Read the model definition and answer for the solid it produces. Units are mm, in the model's axes. A direction names the side the tool comes from. Give positions to 0.01 mm unless a question says otherwise; leave off trailing zeros. Loops run counter-clockwise (first coordinate to the right, second up) from the corner with the lowest first, then second, coordinate; pieces in that order, holes last. Notation, with made-up numbers: (15.25, 23) - (52.25, 23) arc R18 ccw to (52.25, 58) - close; hole circle Ø3 at (57.5, 44). An arc over 180 degrees is marked (long way). Put each result on its own line as item: value. Start each with the question number.
1. Given pin 1 Ø12 at (x, z) = (-4.5, 12) entering from -Y; pin 2 Ø4 at (x, z) = (-8.5, 9.5) entering from -Y; pin 3 Ø5 at (y, z) = (6, 8) entering from +X; pin 4 Ø2 at (x, y) = (37.5, -1.5) entering from -Z, each flat-ended and moving along its own axis, determine where each tip first touches the part or whether it passes through.
2. For a pull along Z with two mould halves and no side action, classify faces 1 (the cylindrical face through (0.426, -1.475, 1.872)), 2 (the cylindrical face through (20.06, 7.95, 8.37)), 3 (the flat face through (-50.8, 0, -5)) as released by +Z, released by -Z, zero draft, split by the parting line, or undercut.
3. A cutting plane is placed at D-D, the plane x = 0. Determine the outline of the cut face in (y, z) (3 decimals), plus the area to 3 significant figures.
4. Consider L1, parallel to Z at x = -18.4, y = 7.75; L2, parallel to X at y = -2.5, z = -4; L3, parallel to Z at x = -30.5, y = -8.5. Determine where each line is inside the solid, lowest interval first. Write a range as from..to.
5. For faces 4 (the cylindrical face through (-47.793, 10.01, -4.998)), 5 (the cylindrical face through (47.793, 10.01, -4.998)), 6 (the flat face through (-25.4, 7, 10)), determine the directions among +Z, -Z, +X, -X, +Y, -Y from which every point of the face is accessible in a straight line to the end or side of a thin tool.
6. A cutting plane is placed at B-B, the plane y = 0. Determine the outline of the cut face in (x, z) (3 decimals), plus the area to 3 significant figures.
7. A cutting plane is placed at C-C, the plane z = 8. Determine the outline of the cut face in (x, y) (3 decimals), plus the area to 3 significant figures.
8. A cutting plane is placed at A-A, the plane x = 38.1. Determine the outline of the cut face in (y, z) (3 decimals), plus the area to 3 significant figures.
```python
from build123d import *

# Parameters (mm, degrees)
SKETCH1_W                = 101.6
SKETCH1_H                = 25.4
BOSS_EXTRUDE1_DEPTH      = 10
SKETCH4_W                = 50.8
SKETCH4_H                = 20
BOSS_EXTRUDE2_DEPTH      = 10
BOSS_EXTRUDE4_DEPTH      = 50.8
BOSS_EXTRUDE4_DEPTH_BACK = 50.8
SKETCH9_W                = 25.4
SKETCH9_H                = 20
CUT_EXTRUDE4_DEPTH       = 61.214616166
FILLET1_R                = 10
CUT_EXTRUDE1_REACH       = 58.726
SKETCH5_R                = 3.175
SKETCH5_R_2              = 1.7
CUT_EXTRUDE2_REACH       = 58.283
SKETCH6_R                = 3.175
FILLET2_R                = 10
CUT_EXTRUDE3_REACH       = 58.726
SKETCH7_R                = 6
SKETCH7_R_2              = 3
FILLET3_R                = 5
FILLET4_R                = 5


with BuildPart() as part:
    # Sketch1 → Boss-Extrude1 (new body)
    with BuildSketch(Plane.XY):
        Rectangle(SKETCH1_W, SKETCH1_H)
    extrude(amount=-BOSS_EXTRUDE1_DEPTH)

    # Sketch4 → Boss-Extrude2 (add)
    with BuildSketch(Plane(origin=(0, 12.7, 0), x_dir=(1, 0, 0), z_dir=(0, 1, 0))):
        with Locations((0, -10)):
            Rectangle(SKETCH4_W, SKETCH4_H)
    extrude(amount=-BOSS_EXTRUDE2_DEPTH)

    # Sketch8 → Boss-Extrude4 (add, two sides: drawn at the far end of the back side and taken through both)
    with BuildSketch(Plane(origin=(0, 0, 0), x_dir=(0, 0, -1), z_dir=(1, 0, 0)).offset(-BOSS_EXTRUDE4_DEPTH_BACK)):
        Polygon((10, 12.7), (-20, 13.680158925), (-20, 12.7), align=None)
    extrude(amount=BOSS_EXTRUDE4_DEPTH + BOSS_EXTRUDE4_DEPTH_BACK)

    # Sketch9 → Cut-Extrude4 (cut, through all)
    with BuildSketch(Plane.XZ.offset(-12.7)):
        with Locations((-38.1, 10)):
            Rectangle(SKETCH9_W, SKETCH9_H)
        with Locations((38.1, 10)):
            Rectangle(SKETCH9_W, SKETCH9_H)
    extrude(amount=-CUT_EXTRUDE4_DEPTH, mode=Mode.SUBTRACT)

    # Fillet1
    fillet1_edges = [part.edges().sort_by_distance(p)[0] for p in [
        (0, 2.7, 0),
    ]]
    fillet(fillet1_edges, radius=FILLET1_R)

    # Cut-Extrude1: up to this plane
    cut_extrude1_end = Plane(origin=(50.8, 12.7, -10), z_dir=(0, -0.9994666982985511, 0.03265454014671021))
    # Sketch5 → Cut-Extrude1 (cut, up to the surface)
    with BuildSketch(Plane(origin=(0, 2.7, 0), x_dir=(1, 0, 0), z_dir=(0, 1, 0)), mode=Mode.PRIVATE) as cut_extrude1_sk1:
        with Locations(Location((0, -8, 0), (0, 0, 90))):
            Circle(SKETCH5_R)
    cut_extrude1_tool1 = split(extrude(cut_extrude1_sk1.sketch, amount=CUT_EXTRUDE1_REACH, mode=Mode.PRIVATE), bisect_by=cut_extrude1_end, keep=Keep.BOTH, mode=Mode.PRIVATE)
    add(cut_extrude1_tool1.solids().sort_by_distance((0, 2.7, 8))[0], mode=Mode.SUBTRACT)
    # Sketch5 → Cut-Extrude1 (cut, up to the surface)
    with BuildSketch(Plane(origin=(0, 2.7, 0), x_dir=(1, 0, 0), z_dir=(0, 1, 0)), mode=Mode.PRIVATE) as cut_extrude1_sk2:
        with Locations(Location((-18.4, -8, 0), (0, 0, 90))):
            Circle(SKETCH5_R_2)
    cut_extrude1_tool2 = split(extrude(cut_extrude1_sk2.sketch, amount=CUT_EXTRUDE1_REACH, mode=Mode.PRIVATE), bisect_by=cut_extrude1_end, keep=Keep.BOTH, mode=Mode.PRIVATE)
    add(cut_extrude1_tool2.solids().sort_by_distance((-18.4, 2.7, 8))[0], mode=Mode.SUBTRACT)
    # Sketch5 → Cut-Extrude1 (cut, up to the surface)
    with BuildSketch(Plane(origin=(0, 2.7, 0), x_dir=(1, 0, 0), z_dir=(0, 1, 0)), mode=Mode.PRIVATE) as cut_extrude1_sk3:
        with Locations(Location((18.4, -8, 0), (0, 0, 90))):
            Circle(SKETCH5_R_2)
    cut_extrude1_tool3 = split(extrude(cut_extrude1_sk3.sketch, amount=CUT_EXTRUDE1_REACH, mode=Mode.PRIVATE), bisect_by=cut_extrude1_end, keep=Keep.BOTH, mode=Mode.PRIVATE)
    add(cut_extrude1_tool3.solids().sort_by_distance((18.4, 2.7, 8))[0], mode=Mode.SUBTRACT)

    # Sketch6 → Cut-Extrude2 (cut, up to next)
    with BuildSketch(Plane.XY, mode=Mode.PRIVATE) as cut_extrude2_sk1:
        with Locations((-38.1, 0)):
            Circle(SKETCH6_R)
    cut_extrude2_tool1 = extrude(cut_extrude2_sk1.sketch, amount=-CUT_EXTRUDE2_REACH, mode=Mode.PRIVATE) & part.part
    # Sketch6 → Cut-Extrude2 (cut, up to next)
    with BuildSketch(Plane.XY, mode=Mode.PRIVATE) as cut_extrude2_sk2:
        with Locations(Location((38.1, 0, 0), (0, 0, 180))):
            Circle(SKETCH6_R)
    cut_extrude2_tool2 = extrude(cut_extrude2_sk2.sketch, amount=-CUT_EXTRUDE2_REACH, mode=Mode.PRIVATE) & part.part
    add(cut_extrude2_tool1.solids().sort_by_distance((-38.1, 0, 0))[0], mode=Mode.SUBTRACT)
    add(cut_extrude2_tool2.solids().sort_by_distance((38.1, 0, 0))[0], mode=Mode.SUBTRACT)

    # Fillet2
    fillet2_edges = [part.edges().sort_by_distance(p)[0] for p in [
        (-50.8, 12.863359821, -5),
        (50.8, 12.863359821, -5),
        (50.8, -12.7, -5),
        (-50.8, -12.7, -5),
    ]]
    fillet(fillet2_edges, radius=FILLET2_R)

    # Sketch7 → Cut-Extrude3 (cut, up to next)
    with BuildSketch(Plane.XZ.offset(-2.7), mode=Mode.PRIVATE) as cut_extrude3_sk1:
        with Locations((0, 8)):
            Circle(SKETCH7_R)
    cut_extrude3_tool1 = extrude(cut_extrude3_sk1.sketch, amount=CUT_EXTRUDE3_REACH, mode=Mode.PRIVATE) & part.part
    # Sketch7 → Cut-Extrude3 (cut, up to next)
    with BuildSketch(Plane.XZ.offset(-2.7), mode=Mode.PRIVATE) as cut_extrude3_sk2:
        with Locations((-18.4, 8)):
            Circle(SKETCH7_R_2)
    cut_extrude3_tool2 = extrude(cut_extrude3_sk2.sketch, amount=CUT_EXTRUDE3_REACH, mode=Mode.PRIVATE) & part.part
    # Sketch7 → Cut-Extrude3 (cut, up to next)
    with BuildSketch(Plane.XZ.offset(-2.7), mode=Mode.PRIVATE) as cut_extrude3_sk3:
        with Locations((18.4, 8)):
            Circle(SKETCH7_R_2)
    cut_extrude3_tool3 = extrude(cut_extrude3_sk3.sketch, amount=CUT_EXTRUDE3_REACH, mode=Mode.PRIVATE) & part.part
    add(cut_extrude3_tool1.solids().sort_by_distance((0, 2.7, 8))[0], mode=Mode.SUBTRACT)
    add(cut_extrude3_tool2.solids().sort_by_distance((-18.4, 2.7, 8))[0], mode=Mode.SUBTRACT)
    add(cut_extrude3_tool3.solids().sort_by_distance((18.4, 2.7, 8))[0], mode=Mode.SUBTRACT)

    # Fillet3
    fillet3_edges = [part.edges().sort_by_distance(p)[0] for p in [
        (-25.4, 2.863359821, 0),
        (25.4, 2.863359821, 0),
    ]]
    fillet(fillet3_edges, radius=FILLET3_R)

    # Fillet4
    fillet4_edges = [part.edges().sort_by_distance(p)[0] for p in [
        (-25.4, 8.190079462, 20),
        (25.4, 8.190079462, 20),
    ]]
    fillet(fillet4_edges, radius=FILLET4_R)


solid = part.part
```
Return value:
1. pin 1: stops at y = 1.92
1. pin 2: stops at y = 2.38
1. pin 3: stops at x = 25.4
1. pin 4: passes through
2. face 1: released by +Z
2. face 2: undercut
2. face 3: zero draft
3. outline: (-12.7, -10) - (12.7, -10) - (13.184, 4.825) - (2.7, 4.825) - (2.7, 2) - (-1.3, 2) arc R10 cw to (-7.3, 0) - (-12.7, 0) - close; (2.7, 11.175) - (13.392, 11.175) - (13.68, 20) - (2.7, 20) - close
3. area: 413 mm2
4. L1: z = -10..6.3, 9.7..20
4. L2: x = -50.8..-40.06, -36.14..36.14, 40.06..50.8
4. L3: z = -10..0
5. face 4: -Z, -X, +Y
5. face 5: -Z, +X, +Y
5. face 6: +Z, -X, +Y, -Y
6. outline: (-50.8, -10) - (-41.275, -10) - (-41.275, 0) - (-50.8, 0) - close; (-34.925, -10) - (34.925, -10) - (34.925, 0) - (30.4, 0) arc R5 cw to (25.749, 3.166) - (3.554, 3.166) arc R6 cw to (-3.554, 3.166) - (-25.749, 3.166) arc R5 cw to (-30.4, 0) - (-34.925, 0) - close; (41.275, -10) - (50.8, -10) - (50.8, 0) - (41.275, 0) - close
6. area: 1,050 mm2
7. outline: (-25.4, 2.498) - (-21.4, 2.498) - (-21.4, 2.7) - (-20.1, 2.7) - (-20.1, 13.288) - (-25.4, 13.288) - close; (-16.7, 2.7) - (-15.4, 2.7) - (-15.4, 2.498) - (-6, 2.498) - (-6, 2.7) - (-3.175, 2.7) - (-3.175, 13.288) - (-16.7, 13.288) - close; (3.175, 2.7) - (6, 2.7) - (6, 2.498) - (15.4, 2.498) - (15.4, 2.7) - (16.7, 2.7) - (16.7, 13.288) - (3.175, 13.288) - close; (20.1, 2.7) - (21.4, 2.7) - (21.4, 2.498) - (25.4, 2.498) - (25.4, 13.288) - (20.1, 13.288) - close
7. area: 404 mm2
8. outline: (-12.7, -10) - (-3.175, -10) - (-3.175, 0) - (-12.7, 0) - close; (3.175, -10) - (12.7, -10) - (13.027, 0) - (3.175, 0) - close
8. area: 192 mm2
